Print and shaded views of the part. All mm, measured from the part's lowest x, y and z. Round coordinates to 2 decimals unless told otherwise and drop trailing zeros. Write each loop counter-clockwise with the first axis right and the second up, starting at its lowest first coordinate (ties: lowest second). Pieces come first, ordered by that corner, then holes. Notation, with made-up numbers: (82.5, 34) - (87.5, 34) arc R24 cw to (87.5, 55) - close; hole circle Ø11 at (-38.5, -34.5). An arc over 180 degrees is marked (long way). Put each result on its own line as item: value. Start each with the question number.
Item 1: Cut at B-B (y = 47.5). Give the cut face in (x, z).
Item 2: Pin check, flat tips, straight feed: pin 1 Ø0.8 at (y, z) = (17, 2) entering from +X; pin 2 Ø1.4 at (y, z) = (76.5, 1.5) entering from -X; pin 3 Ø0.8 at (x, z) = (164.5, 2) entering from +Y; pin 4 Ø1.4 at (x, z) = (1.5, 1.5) entering from -Y. Stop position of each tip, or through.
Item 3: Drill centre lines: line 1 (Y direction, x = 82.7, z = 1.15) (1 decimal); line 2 (X direction, y = 47.5, z = 1.9); line 3 (X direction, y = 75.5, z = 0.15). Where is each one in solid material? Low to high. Write a range as from..to.
Item 4: Cut at A-A (x = 82.7). Give the cut face in (y, z) (1 decimal).
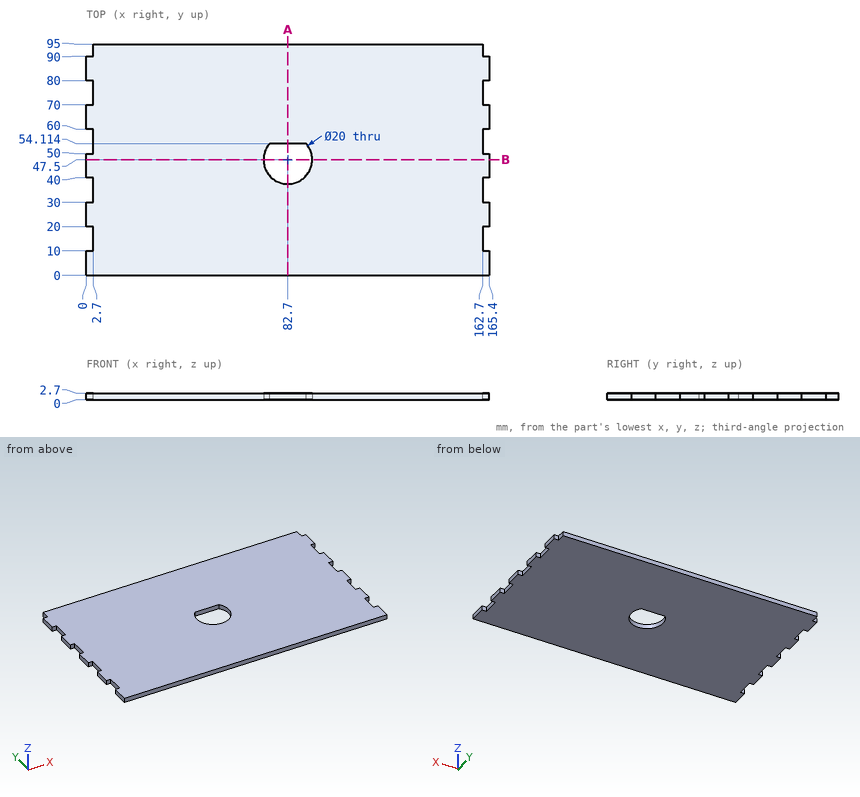
Output values:
1. outline: (0, 0) - (72.7, 0) - (72.7, 2.7) - (0, 2.7) - close; (92.7, 0) - (165.4, 0) - (165.4, 2.7) - (92.7, 2.7) - close
2. pin 1: x = 162.7
2. pin 2: x = 2.7
2. pin 3: y = 90
2. pin 4: y = 0
3. line 1: 0..37.5, 54.1..95
3. line 2: 0..72.7, 92.7..165.4
3. line 3: 2.7..162.7
4. outline: (0, 0) - (37.5, 0) - (37.5, 2.7) - (0, 2.7) - close; (54.1, 0) - (95, 0) - (95, 2.7) - (54.1, 2.7) - close
